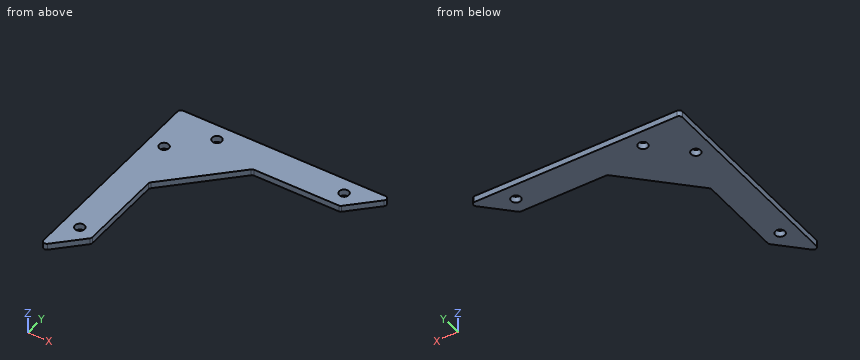
from build123d import *

# Parameters (mm, degrees)
SKETCH_R  = 3
PAD_DEPTH = 4


with BuildPart() as part:
    # Sketch → Pad (new body)
    with BuildSketch(Plane.XY):
        with BuildLine():
            Line((2, 0), (129.313708, 0))
            ThreePointArc((130.727922, -3.414214), (131.161468, -1.234633), (129.313708, 0))
            Line((114.727922, -19.414214), (130.727922, -3.414214))
            ThreePointArc((113.313708, -20), (114.079075, -19.847759), (114.727922, -19.414214))
            Line((113.313708, -20), (60, -20))
            ThreePointArc((60, -20), (59.234633, -20.152241), (58.585786, -20.585786))
            Line((58.585786, -20.585786), (20.585786, -58.585786))
            ThreePointArc((20.585786, -58.585786), (20.152241, -59.234633), (20, -60))
            Line((20, -60), (20, -113.313708))
            ThreePointArc((19.414214, -114.727922), (19.847759, -114.079075), (20, -113.313708))
            Line((3.414214, -130.727922), (19.414214, -114.727922))
            ThreePointArc((0, -129.313708), (1.234633, -131.161468), (3.414214, -130.727922))
            Line((0, -129.313708), (0, -2))
            ThreePointArc((2, 0), (0.585786, -0.585786), (0, -2))
        make_face()
        with Locations((10, -110)):
            Circle(SKETCH_R, mode=Mode.SUBTRACT)
        with Locations((110, -10)):
            Circle(SKETCH_R, mode=Mode.SUBTRACT)
        with Locations((10, -30)):
            Circle(SKETCH_R, mode=Mode.SUBTRACT)
        with Locations((30, -10)):
            Circle(SKETCH_R, mode=Mode.SUBTRACT)
    extrude(amount=PAD_DEPTH)


solid = part.part
Read the model definition and answer for the solid it produces. Units are mm, in the model's axes. Give positions to 0.01 mm unless a question says otherwise; leave off trailing zeros. Write each loop counter-clockwise with the first axis right and the second up, starting at its lowest first coordinate (ties: lowest second). Pieces come first, ordered by that corner, then holes. Notation, with made-up numbers: (49, 14.25) - (92, 14.25) arc R11 ccw to (92, 23.25) - close; hole circle Ø8 at (25, -26). An arc over 180 degrees is marked (long way). Answer in a Markdown table with one row per item. Add a question column.
Item 1: Section C-C, the plane x = 110 is taken. Write down the section's boundary in (y, z), and give its area (3 significant figures).
Item 2: Find the intervals of material crossed by L1, parallel to Y at x = 110, z = 2.8; L2, parallel to X at y = -95.5, z = 0.6; L3, parallel to X at y = -31.5, z = 2, in increasing order.
Item 3: Section D-D, the plane y = -10 is taken. Write down the section's boundary in (x, z), and give its area (3 significant figures).
Item 4: Section B-B, the plane z = 2.25 is taken. Write down the section's boundary in (x, y).
Item 5: Section A-A, the plane y = -110 is taken. Write down the section's boundary in (x, z), and give its area (3 significant figures).
Item 6: Flat-ended cylindrical pins translate along their axes: P1, Ø1.2, axis at y = -97.5, z = 1.5, coming from the +X side; P2, Ø2, axis at y = -16, z = 2, coming from the +X side. Find the tip coordinate at first contact, or state that the pin passes through.
Recorded:
| question | item | result |
|---|---|---|
| 1 | outline | (-20, 0) - (-13, 0) - (-13, 4) - (-20, 4) - close; (-7, 0) - (0, 0) - (0, 4) - (-7, 4) - close |
| 1 | area | 56.0 mm2 |
| 2 | L1 | y = -20 to -13, -7 to 0 |
| 2 | L2 | x = 0 to 20 |
| 2 | L3 | x = 0 to 7.4, 12.6 to 47.67 |
| 3 | outline | (0, 0) - (27, 0) - (27, 4) - (0, 4) - close; (33, 0) - (107, 0) - (107, 4) - (33, 4) - close; (113, 0) - (124.14, 0) - (124.14, 4) - (113, 4) - close |
| 3 | area | 449 mm2 |
| 4 | outline | (0, -129.31) arc R2 ccw to (3.41, -130.73) - (19.41, -114.73) arc R2 ccw to (20, -113.31) - (20, -60) arc R2 cw to (20.59, -58.59) - (58.59, -20.59) arc R2 cw to (60, -20) - (113.31, -20) arc R2 ccw to (114.73, -19.41) - (130.73, -3.41) arc R2 ccw to (129.31, 0) - (2, 0) arc R2 ccw to (0, -2) - close; hole circle Ø6 at (10, -110); hole circle Ø6 at (10, -30); hole circle Ø6 at (30, -10); hole circle Ø6 at (110, -10) |
| 5 | outline | (0, 0) - (7, 0) - (7, 4) - (0, 4) - close; (13, 0) - (20, 0) - (20, 4) - (13, 4) - close |
| 5 | area | 56.0 mm2 |
| 6 | P1 | stops at x = 20 |
| 6 | P2 | stops at x = 119.14 |
